Check sheet for the modelled part. Datum: model origin and axes. Units: mm. Face numbers are marked on the shaded views. A direction names the side the tool comes from. Coordinates: 2 decimals unless noted, no trailing zeros. Loops run counter-clockwise (first coordinate to the right, second up) from the corner with the lowest first, then second, coordinate; pieces in that order, holes last.
Autodesk Inventor part; units mm, degrees
ref_plane "rod_cp_XY" through (0, 0, 0) normal (1, 0, 0) x (0, 0, -1)
ref_plane "rod_cp_YZ" through (0, 0, 0) normal (0, 0, -1) x (0, 1, 0)
ref_plane "rod_cp_ZX" through (0, 0, 0) normal (0, 1, 0) x (1, 0, 0)
sketch "Sketch_1" plane through (0, 0, 0) normal (0, 0, 1) x (1, 0, 0)
  line L0 (150.8506, 0) -> (0, 0)
  line L1 (0, 0) -> (0, 3.175)
  line L2 (0, 3.175) -> (129.3876, 3.175)
  line L3 (129.3876, 3.175) -> (129.3876, 9.6203)
  line L4 (129.3876, 9.6203) -> (150.8506, 9.6203)
  line L5 (150.8506, 9.6203) -> (150.8506, 0)
  line L6 (150.8506, 0) -> (0, 0)
revolve "Revolution1" add sketch "Sketch_1" angle 360 about axis through (150.8506, 0, 0) along (1, 0, 0)
sketch "Sketch_3" plane through (0, 0, 0) normal (0, 0, 1) x (1, 0, 0)
  line L0 (0, 0) -> (-12.7, 0)
  line L1 (-12.7, 0) -> (-12.7, 2.634)
  line L2 (-12.7, 2.634) -> (-12.159, 3.175)
  line L3 (-12.159, 3.175) -> (0, 3.175)
  line L4 (0, 3.175) -> (0, 0)
  line L5 (0, 0) -> (-12.7, 0)
revolve "Revolution2" add sketch "Sketch_3" angle 360 about axis through (0, 0, 0) along (1, 0, 0)
thread "Thread1"
sketch "Sketch_30" plane through (0, 0, 0) normal (0, 0, 1) x (1, 0, 0)
  line L0 (0, 0) -> (-0.254, 0)
  line L1 (-0.254, 3.429) -> (-0.254, 2.921)
  line L2 (-0.254, 2.921) -> (0, 2.921)
  line L3 (0, 2.921) -> (0, 3.429)
  line L4 (0, 3.429) -> (-0.254, 3.429)
revolve "Revolution3" cut sketch "Sketch_30" angle 360 about axis through (0, 0, 0) along (1, 0, 0)
ref_plane "rod_cp_XY" through (0, 0, 0) normal (1, 0, 0) x (0, 0, -1)
ref_plane "rod_cp_YZ" through (0, 0, 0) normal (0, 0, -1) x (0, 1, 0)
ref_plane "rod_cp_ZX" through (0, 0, 0) normal (0, 1, 0) x (1, 0, 0)
ref_plane "to_rod_clevis_XY" through (-12.7, 0, 0) normal (1, 0, 0) x (0, 0, -1)
ref_plane "to_rod_clevis_YZ" through (-12.7, 0, 0) normal (0, 0, -1) x (0, 1, 0)
ref_plane "to_rod_clevis_ZX" through (-12.7, 0, 0) normal (0, 1, 0) x (1, 0, 0)
ref_plane "rl2_XY" through (0, 0, 0) normal (1, 0, 0) x (0, 0, -1)
ref_plane "rl2_YZ" through (0, 0, 0) normal (0, 0, -1) x (0, 1, 0)
ref_plane "rl2_ZX" through (0, 0, 0) normal (0, 1, 0) x (1, 0, 0)
ref_plane "rl1_XY" through (-12.7, 0, 0) normal (1, 0, 0) x (0, 0, -1)
ref_plane "rl1_YZ" through (-12.7, 0, 0) normal (0, 0, -1) x (0, 1, 0)
ref_plane "rl1_ZX" through (-12.7, 0, 0) normal (0, 1, 0) x (1, 0, 0)
ref_plane "thd1_XY" through (-12.7, 3.175, 0) normal (1, 0, 0) x (0, 0, -1)
ref_plane "thd1_YZ" through (-12.7, 3.175, 0) normal (0, 0, -1) x (0, 1, 0)
ref_plane "thd1_ZX" through (-12.7, 3.175, 0) normal (0, 1, 0) x (1, 0, 0)
ref_plane "thd2_XY" through (-12.7, -3.175, 0) normal (1, 0, 0) x (0, 0, -1)
ref_plane "thd2_YZ" through (-12.7, -3.175, 0) normal (0, 0, -1) x (0, 1, 0)
ref_plane "thd2_ZX" through (-12.7, -3.175, 0) normal (0, 1, 0) x (1, 0, 0)
ref_plane "dia1_XY" through (0, 3.175, 0) normal (1, 0, 0) x (0, 0, -1)
ref_plane "dia1_YZ" through (0, 3.175, 0) normal (0, 0, -1) x (0, 1, 0)
ref_plane "dia1_ZX" through (0, 3.175, 0) normal (0, 1, 0) x (1, 0, 0)
ref_plane "dia2_XY" through (0, -3.175, 0) normal (1, 0, 0) x (0, 0, -1)
ref_plane "dia2_YZ" through (0, -3.175, 0) normal (0, 0, -1) x (0, 1, 0)
ref_plane "dia2_ZX" through (0, -3.175, 0) normal (0, 1, 0) x (1, 0, 0)
ref_plane "dia1r_XY" through (0, 0, 10.2235) normal (1, 0, 0) x (0, 0, -1)
ref_plane "dia1r_YZ" through (0, 0, 10.2235) normal (0, 0, -1) x (0, 1, 0)
ref_plane "dia1r_ZX" through (0, 0, 10.2235) normal (0, 1, 0) x (1, 0, 0)
ref_plane "dia2r_XY" through (0, 0, -10.2235) normal (1, 0, 0) x (0, 0, -1)
ref_plane "dia2r_YZ" through (0, 0, -10.2235) normal (0, 0, -1) x (0, 1, 0)
ref_plane "dia2r_ZX" through (0, 0, -10.2235) normal (0, 1, 0) x (1, 0, 0)
ref_plane "dia12_XY" through (0, 0, 10.9537) normal (1, 0, 0) x (0, 0, -1)
ref_plane "dia12_YZ" through (0, 0, 10.9537) normal (0, 0, -1) x (0, 1, 0)
ref_plane "dia12_ZX" through (0, 0, 10.9537) normal (0, 1, 0) x (1, 0, 0)
ref_plane "dia22_XY" through (0, 0, -10.9537) normal (1, 0, 0) x (0, 0, -1)
ref_plane "dia22_YZ" through (0, 0, -10.9537) normal (0, 0, -1) x (0, 1, 0)
ref_plane "dia22_ZX" through (0, 0, -10.9537) normal (0, 1, 0) x (1, 0, 0)
properties part number "043.5-DQ0_rod"
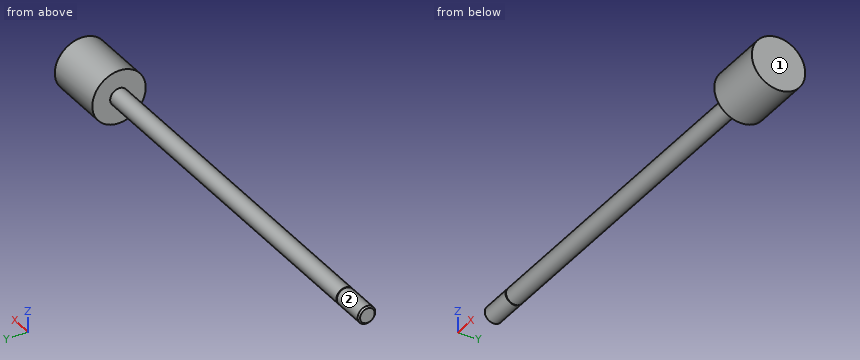
1) Scan lines: line 1 (X direction, y = -7, z = -5.5); line 2 (Y direction, x = 89.5, z = 0.25); line 3 (Z direction, x = 29, y = -1.25). Record each from-to range of solid material in increasing order.
Answer sheet:
line 1: x = 129.39 to 150.85
line 2: y = -3.17 to 3.17
line 3: z = -2.92 to 2.92
2) Section check D-D on z = 7. Enter the section's corners in (x, y).
Answer sheet:
outline: (129.39, -6.6) - (150.85, -6.6) - (150.85, 6.6) - (129.39, 6.6) - close
3) Set-up check for the marked faces 1 and 2: record each of +Z, -Z, +X, -X, +Y, -Y from which the full face is reachable in a straight line by a thin tool's end or side.
Answer sheet:
face 1: +Z, -Z, +X, +Y, -Y
face 2: -X
4) Depth check by flat-ended pin: pin 1 (6 mm diameter, centred on x = 63, z = 0, fed in from -Y) (3 decimals); pin 2 (4 mm diameter, centred on x = 91, z = -1.5, fed in from +Y) (3 decimals); pin 3 (2 mm diameter, centred on x = 96.5, z = -1.5, fed in from -Y). Enter the tip coordinate at first touch or a pass-through.
Answer sheet:
pin 1: stops at y = -3.175
pin 2: stops at y = 3.175
pin 3: stops at y = -3.14
5) Section check A-A on y = 0. Enter the section's corners in (x, z) (3 decimals), plus the area to 3 significant figures.
Answer sheet:
outline: (-12.7, -2.634) - (-12.159, -3.175) - (-0.254, -3.175) - (-0.254, -2.921) - (0, -2.921) - (0, -3.175) - (129.388, -3.175) - (129.388, -9.62) - (150.851, -9.62) - (150.851, 9.62) - (129.388, 9.62) - (129.388, 3.175) - (0, 3.175) - (0, 2.921) - (-0.254, 2.921) - (-0.254, 3.175) - (-12.159, 3.175) - (-12.7, 2.634) - close
area: 1,310 mm2
6) Section check C-C on x = 72. Enter the section's corners in (y, z) (3 decimals), plus the area to 3 significant figures.
Answer sheet:
outline: circle Ø6.35 at (0, 0)
area: 31.7 mm2
